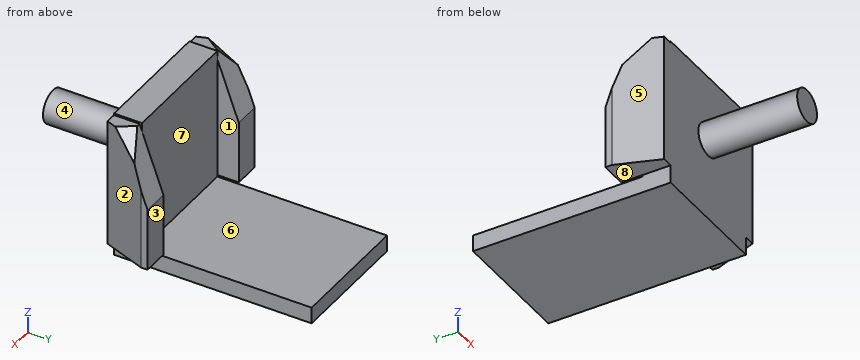
```python
from build123d import *
from OCP.BRepFilletAPI import BRepFilletAPI_MakeChamfer

# Parameters (mm, degrees)
SKETCH1_W           = 380
SKETCH1_H           = 400
BOSS_EXTRUDE1_DEPTH = 85
SKETCH2_W           = 80
SKETCH2_H           = 390
BOSS_EXTRUDE2_DEPTH = 150
CHAMFER1_SIZE       = 72.794046853
CHAMFER1_SIZE_2     = 200
CHAMFER2_SIZE       = 130
CHAMFER2_SIZE2      = 47.316130455
SKETCH3_W           = 380
SKETCH3_H           = 600
BOSS_EXTRUDE3_DEPTH = 50
SKETCH4_R           = 50
BOSS_EXTRUDE4_DEPTH = 300
CHAMFER3_START      = 285.464373586
CHAMFER3_OUTLINE_W  = 79
CHAMFER3_OUTLINE_H  = 106
CHAMFER3_DEPTH      = 30.956619547
CHAMFER4_START      = -316.420993133
CHAMFER4_OUTLINE_W  = 79
CHAMFER4_OUTLINE_H  = 106
CHAMFER4_DEPTH      = 30.956619547


with BuildPart() as part:
    # Sketch1 → Boss-Extrude1 (new body)
    with BuildSketch(Plane(origin=(0, 0, 0), x_dir=(1, 0, 0), z_dir=(0, 1, 0))):
        Rectangle(SKETCH1_W, SKETCH1_H)
    extrude(amount=BOSS_EXTRUDE1_DEPTH)

    # Sketch2 → Boss-Extrude2 (add)
    with BuildSketch(Plane(origin=(0, 0, 0), x_dir=(1, 0, 0), z_dir=(0, 1, 0))):
        with Locations((-230, 0)):
            Rectangle(SKETCH2_W, SKETCH2_H)
        with Locations((230, 0)):
            Rectangle(SKETCH2_W, SKETCH2_H)
    extrude(amount=BOSS_EXTRUDE2_DEPTH)

    # Chamfer1
    # the kernel refuses this chamfer: 200, 72.794046853 mm, written as the material it takes off along each edge
    with BuildSketch(Plane(origin=(-788.83894651, 150, 195), x_dir=(0, -1, 0), z_dir=(1, 0, 0)), Plane(origin=(190, 150, 195), x_dir=(0, -1, 0), z_dir=(1, 0, 0))) as chamfer1_piece_1:
        Polygon((CHAMFER1_SIZE, 0), (0, CHAMFER1_SIZE_2), (0, 0), align=None)
    extrude(amount=598.83894651, mode=Mode.SUBTRACT)
    with BuildSketch(Plane(origin=(-788.83894651, 150, 195), x_dir=(0, -1, 0), z_dir=(1, 0, 0))) as chamfer1_piece_2_section:
        Polygon((CHAMFER1_SIZE, 0), (0, CHAMFER1_SIZE_2), (0, 0), align=None)
    chamfer1_piece_2 = extrude(amount=1117.67789302, mode=Mode.PRIVATE)
    chamfer1_piece_2 = split(chamfer1_piece_2, bisect_by=Plane(origin=(190, 150, 195), z_dir=(1, 0, 0)), keep=Keep.TOP, mode=Mode.PRIVATE)
    add(chamfer1_piece_2, mode=Mode.SUBTRACT)
    with BuildSketch(Plane(origin=(-328.83894651, 150, 195), x_dir=(0, -1, 0), z_dir=(1, 0, 0))) as chamfer1_piece_3_section:
        Polygon((CHAMFER1_SIZE, 0), (0, CHAMFER1_SIZE_2), (0, 0), align=None)
    chamfer1_piece_3 = extrude(amount=1117.67789302, mode=Mode.PRIVATE)
    chamfer1_piece_3 = split(chamfer1_piece_3, bisect_by=Plane(origin=(-190, 150, 195), z_dir=(-1, 0, 0)), keep=Keep.TOP, mode=Mode.PRIVATE)
    add(chamfer1_piece_3, mode=Mode.SUBTRACT)

    # Chamfer2: one chamfer whose edges measure the first distance from different faces: ONE call of the kernel's chamfer builder (chamfer() names one face for all edges)
    chamfer2_edges_1 = [part.edges().sort_by_distance(p)[0] for p in [
        (270, 0, 0),
    ]]
    chamfer2_side_1 = [part.faces().sort_by_distance(p)[0] for p in [
        (270, 67.789562339, -18.238567166),
    ]]
    chamfer2_edges_2 = [part.edges().sort_by_distance(p)[0] for p in [
        (-270, 0, 0),
    ]]
    chamfer2_side_2 = [part.faces().sort_by_distance(p)[0] for p in [
        (-270, 67.789562339, -18.238567166),
    ]]
    chamfer2 = BRepFilletAPI_MakeChamfer(part.part.solid().wrapped)
    for e in chamfer2_edges_1:
        chamfer2.Add(CHAMFER2_SIZE, CHAMFER2_SIZE2, e.wrapped, chamfer2_side_1[0].wrapped)  # the first distance lies on this face
    for e in chamfer2_edges_2:
        chamfer2.Add(CHAMFER2_SIZE, CHAMFER2_SIZE2, e.wrapped, chamfer2_side_2[0].wrapped)  # the first distance lies on this face
    add(Compound.cast(chamfer2.Shape()), mode=Mode.REPLACE)

    # Sketch3 → Boss-Extrude3 (add)
    with BuildSketch(Plane(origin=(0, 0, -200), x_dir=(-1, 0, 0), z_dir=(0, 0, -1))):
        with Locations((0, 300)):
            Rectangle(SKETCH3_W, SKETCH3_H)
    extrude(amount=BOSS_EXTRUDE3_DEPTH)

    # Sketch4 → Boss-Extrude4 (add)
    with BuildSketch(Plane.XZ):
        with Locations(Location((0, 0, 0), (0, 0, 270))):
            Circle(SKETCH4_R)
    extrude(amount=BOSS_EXTRUDE4_DEPTH)

    # Chamfer3: read off the stored shape, not the designer's step
    # Chamfer3 outline → Chamfer3 (cut)
    with BuildSketch(Plane(origin=(0, 0, 0), x_dir=(0.7852866244263759, -0.34179494272055927, -0.5162374789064406), z_dir=(0.6191323909286511, 0.433521167278043, 0.6547781914701)).offset(CHAMFER3_START)):
        with Locations((68.5, -31)):
            Rectangle(CHAMFER3_OUTLINE_W, CHAMFER3_OUTLINE_H)
    extrude(amount=CHAMFER3_DEPTH, mode=Mode.SUBTRACT)

    # Chamfer4: read off the stored shape, not the designer's step
    # Chamfer4 outline → Chamfer4 (cut)
    with BuildSketch(Plane(origin=(0, 0, 0), x_dir=(0.7852866244263759, 0.34179494272055927, 0.5162374789064406), z_dir=(0.6191323909286511, -0.433521167278043, -0.6547781914701)).offset(CHAMFER4_START)):
        with Locations((-68.5, 31)):
            Rectangle(CHAMFER4_OUTLINE_W, CHAMFER4_OUTLINE_H)
    extrude(amount=CHAMFER4_DEPTH, mode=Mode.SUBTRACT)


solid = part.part
```
Check sheet for the modelled part. Datum: model origin and axes. Units: mm. Face numbers are marked on the shaded views. A direction names the side the tool comes from. Give positions to 0.01 mm unless a question says otherwise; leave off trailing zeros. Order: outer loops, then holes, each group sorted by start corner. A loop starts at its lowest first (then second) coordinate and runs counter-clockwise, first axis right, second up. Notation, with made-up numbers: M 69.25,61 L 103.25,61 A18 cw 103.25,95 Z; hole C 67.5,-15.5 d4. An arc over 180 degrees is marked long. Answer in a Markdown table with one row per item. Add a question column.
Q1. Gauge pin test, flat ends, axial feed: pin 1 Ø1.5 at (x, y) = (-112, 182) entering from +Z; pin 2 Ø24 at (x, z) = (-225, -60) entering from +Y; pin 3 Ø3 at (x, y) = (-190.5, 354.5) entering from -Z; pin 4 Ø8 at (y, z) = (-112.5, 10) entering from +X. Record the tip position at first contact, or that the pin passes through.
Q2. Thickness scan on L1, parallel to Z at x = -94, y = 387; L2, parallel to Y at x = 28.5, z = -205.5; L3, parallel to Y at x = 46.5, z = 69.5. Record the ranges inside material, lowest first.
Q3. Sectioned sample at D-D, the plane x = 128. Record the boundary of the cut face in (y, z).
Q4. Sectioned sample at B-B, the plane z = -106. Record the boundary of the cut face in (x, y), and give its area (3 significant figures).
Q5. Sectioned sample at C-C, the plane y = 231. Record the boundary of the cut face in (x, z), and give its area (3 significant figures).
Q6. Access from +Z, -Z, +X, -X, +Y, -Y to the whole of each face (thin tool, end or side, straight path). Record for the marked faces 4, 5, 6, 7 and 8.
Q7. Sectioned sample at A-A, the plane x = 0. Record the boundary of the cut face in (y, z), and give its area (3 significant figures).
Q8. Release check for a two-part mould opening along X. For the marked faces 1, 2 and 3 record: released by +X, released by -X, zero draft, split by the parting line, or undercut.
Verdict:
| question | item | result |
|---|---|---|
| 1 | pin 1 | z = -200 |
| 1 | pin 2 | y = 150 |
| 1 | pin 3 | z = -250 |
| 1 | pin 4 | x = 49.64 |
| 2 | L1 | -250 to -200 |
| 2 | L2 | 0 to 600 |
| 2 | L3 | 0 to 85 |
| 3 | outline | M 0,-250 L 600,-250 L 600,-200 L 85,-200 L 85,200 L 0,200 Z |
| 4 | outline | M -270,130 L -222.68,0 L 222.68,0 L 270,130 L 270,150 L 190,150 L 190,85 L -190,85 L -190,150 L -270,150 Z |
| 4 | area | 50,100 mm² |
| 5 | outline | M -190,-250 L 190,-250 L 190,-200 L -190,-200 Z |
| 5 | area | 19,000 mm² |
| 6 | face 4 | -Y |
| 6 | face 5 | +Z, -Z, -X, -Y |
| 6 | face 6 | +Z, +X, -X, +Y |
| 6 | face 7 | +Z, +Y |
| 6 | face 8 | -Z, -X, +Y, -Y |
| 7 | outline | M -300,-50 L 0,-50 L 0,-250 L 600,-250 L 600,-200 L 85,-200 L 85,200 L 0,200 L 0,50 L -300,50 Z |
| 7 | area | 94,000 mm² |
| 8 | face 1 | undercut |
| 8 | face 2 | released by +X |
| 8 | face 3 | zero draft |
